Verification items for the finished model (mm, model axes). A direction names the side the tool comes from. Round coordinates to 2 decimals unless told otherwise and drop trailing zeros. Write each loop counter-clockwise with the first axis right and the second up, starting at its lowest first coordinate (ties: lowest second). Pieces come first, ordered by that corner, then holes.
from build123d import *

# Parameters (mm, degrees)
SKETCH_1_R      = 2.05
SKETCH_1_R_2    = 1.6
EXTRUDE_1_DEPTH = 4
FILLET_1_R      = 2
CHAMFER_1_SIZE  = 1.5
FILLET_2_R      = 2


with BuildPart() as part:
    # Эскиз1 → Бобышка-Вытянуть1 (new body)
    with BuildSketch(Plane.XY):
        Polygon((0, 8), (0, 0), (5.75, 0), (5.75, -4), (45.75, -4), (45.75, 0), (51.5, 0), (51.5, 8), (45.75, 8), (45.75, 22), (5.75, 22), (5.75, 8), align=None)
        with Locations((12.75, 4)):
            Circle(SKETCH_1_R, mode=Mode.SUBTRACT)
        with Locations((4, 4)):
            Circle(SKETCH_1_R_2, mode=Mode.SUBTRACT)
        with BuildLine():
            ThreePointArc((27.85, 4), (25.75, 1.9), (23.65, 4))
            ThreePointArc((23.65, 4), (25.75, 6.1), (27.85, 4))
        make_face(mode=Mode.SUBTRACT)
        with Locations((38.75, 4)):
            Circle(SKETCH_1_R, mode=Mode.SUBTRACT)
        with Locations((47.5, 4)):
            Circle(SKETCH_1_R_2, mode=Mode.SUBTRACT)
    extrude(amount=EXTRUDE_1_DEPTH)

    # Скругление1
    fillet_1_edges = [part.edges().sort_by_distance(p)[0] for p in [
        (0, 0, 2),
        (0, 8, 2),
        (51.5, 8, 2),
        (51.5, 0, 2),
    ]]
    fillet(fillet_1_edges, radius=FILLET_1_R)

    # Фаска1
    chamfer_1_edges = [part.edges().sort_by_distance(p)[0] for p in [
        (2.4, 4, 4),
        (45.9, 4, 4),
    ]]
    chamfer(chamfer_1_edges, length=CHAMFER_1_SIZE)

    # Скругление2
    fillet_2_edges = [part.edges().sort_by_distance(p)[0] for p in [
        (5.75, 22, 2),
        (45.75, 22, 2),
        (45.75, -4, 2),
        (5.75, -4, 2),
    ]]
    fillet(fillet_2_edges, radius=FILLET_2_R)


solid = part.part
Q1. Material ranges on line 1 along Y through (x, z) = (25.75, 2.2); line 2 along Y through (x, z) = (38.75, 2.6); line 3 along X through (y, z) = (3.5, 0.6), recorded low to high.
Recorded:
line 1: y = -4 to 1.9, 6.1 to 22
line 2: y = -4 to 1.95, 6.05 to 22
line 3: x = 0 to 2.48, 5.52 to 10.76, 14.74 to 23.71, 27.79 to 36.76, 40.74 to 45.98, 49.02 to 51.5
Q2. Tool access check on faces 4 (the flat face through (5.75, -1, 2)), 5 (the flat face through (45.75, 14, 2)), 6 (the flat face through (4, 8, 2)), 7 (the cylindrical face through (5.48, 3.39, 1.23)), 8 (the flat face through (48, 0, 2)). Record the directions out of +Z, -Z, +X, -X, +Y, -Y that give a thin tool (end or side, any length) a straight path to the whole face; none if there is none.
Recorded:
face 4: +Z, -Z, -X, -Y
face 5: +Z, -Z, +X, +Y
face 6: +Z, -Z, -X, +Y
face 7: +Z, -Z
face 8: +Z, -Z, +X, -Y
Q3. Sectioned sample at B-B (z = 3.4). Enter the section's corners in (x, y).
Recorded:
outline: (0, 2) arc R2 ccw to (2, 0) - (5.75, 0) - (5.75, -2) arc R2 ccw to (7.75, -4) - (43.75, -4) arc R2 ccw to (45.75, -2) - (45.75, 0) - (49.5, 0) arc R2 ccw to (51.5, 2) - (51.5, 6) arc R2 ccw to (49.5, 8) - (45.75, 8) - (45.75, 20) arc R2 ccw to (43.75, 22) - (7.75, 22) arc R2 ccw to (5.75, 20) - (5.75, 8) - (2, 8) arc R2 ccw to (0, 6) - close; hole circle Ø5 at (4, 4); hole circle Ø4.1 at (12.75, 4); hole circle Ø4.2 at (25.75, 4); hole circle Ø4.1 at (38.75, 4); hole circle Ø5 at (47.5, 4)
Q4. Sectioned sample at D-D (y = 4.5). Give the number of separate pieces and of enclosed holes in the cut face, plus the area to 3 significant figures.
Recorded:
separate pieces: 6
enclosed holes: 0
area: 129 mm2
Q5. Release check for a two-part mould opening along X. For faces 1 (the cylindrical face through (49.026, 4.481, 1.232)), 2 (the cylindrical face through (6.32, -3.4, 2.03)), 3 (the cylindrical face through (50.9, 7.43, 2.03)) record: released by +X, released by -X, zero draft, split by the parting line, or undercut.
Recorded:
face 1: undercut
face 2: released by -X
face 3: released by +X
Q6. Sectioned sample at C-C (x = 47.5). Enter the section's corners in (y, z), plus the area to 4 significant figures.
Recorded:
outline: (0, 0) - (2.4, 0) - (2.4, 2.5) - (0.9, 4) - (0, 4) - close; (5.6, 0) - (8, 0) - (8, 4) - (7.1, 4) - (5.6, 2.5) - close
area: 16.95 mm2
Q7. Sectioned sample at A-A (x = 25.75). Enter the section's corners in (y, z).
Recorded:
outline: (-4, 0) - (1.9, 0) - (1.9, 4) - (-4, 4) - close; (6.1, 0) - (22, 0) - (22, 4) - (6.1, 4) - close
Q8. Depth check by flat-ended pin: P1, Ø2, axis at y = 17.5, z = 0.5, coming from the -X side; P2, Ø1.1, axis at x = 47.5, z = 1, coming from the +Y side; P3, Ø6.5, axis at x = 25.75, y = 4, coming from the -Z side; P4, Ø0.6, axis at y = -1, z = 3, coming from the +X side. Enter the tip coordinate at first touch or a pass-through.
Recorded:
P1: stops at x = 5.75
P2: stops at y = 8
P3: stops at z = 0
P4: stops at x = 45.75
